```python
from build123d import *

# Parameters (mm, degrees)
BOSS_EXTRUDE1_DEPTH = 8
SKETCH2_W           = 23.137445614
SKETCH2_H           = 10.306738945
BOSS_EXTRUDE2_DEPTH = 8
SKETCH4_W           = 1
SKETCH4_H           = 2
CUT_EXTRUDE1_DEPTH  = 60
FILLET1_R           = 0.5


with BuildPart() as part:
    # Sketch1 → Boss-Extrude1 (new body)
    with BuildSketch(Plane(origin=(0, 0, 0), x_dir=(1, 0, 0), z_dir=(0, 1, 0))):
        with BuildLine():
            Line((11.568722807, -17.464704369), (11.568722807, 17.464704369))
            Line((11.568722807, 17.464704369), (0, 17.464704369))
            Line((0, 17.464704369), (0, -2.002357687))
            ThreePointArc((0, -2.002357687), (4.242640687, -3.759717), (6, -8.002357687))
            ThreePointArc((6, -8.002357687), (4.242640687, -12.244998375), (0, -14.002357687))
            Line((0, -14.002357687), (0, -17.464704369))
            Line((0, -17.464704369), (11.568722807, -17.464704369))
        make_face()
        with BuildLine():
            Line((0, -2.002357687), (0, 17.464704369))
            Line((0, 17.464704369), (-11.568722807, 17.464704369))
            Line((-11.568722807, 17.464704369), (-11.568722807, -17.464704369))
            Line((-11.568722807, -17.464704369), (0, -17.464704369))
            Line((0, -17.464704369), (0, -14.002357687))
            ThreePointArc((0, -14.002357687), (-6, -8.002357687), (0, -2.002357687))
        make_face()
    extrude(amount=BOSS_EXTRUDE1_DEPTH)

    # Sketch2 → Boss-Extrude2 (add)
    with BuildSketch(Plane.XZ):
        with Locations((0, -22.618073841)):
            Rectangle(SKETCH2_W, SKETCH2_H)
    extrude(amount=-BOSS_EXTRUDE2_DEPTH)

    # Sketch4 → Cut-Extrude1 (cut)
    with BuildSketch(Plane(origin=(11.568722807, 0, 0), x_dir=(0, 0, -1), z_dir=(1, 0, 0))):
        with Locations((13.536168456, 8)):
            Rectangle(SKETCH4_W, SKETCH4_H)
    extrude(amount=-CUT_EXTRUDE1_DEPTH, mode=Mode.SUBTRACT)

    # Fillet1
    fillet1_edges = [part.edges().sort_by_distance(p)[0] for p in [
        (0, 7, -14.036168456),
        (0, 7, -13.036168456),
    ]]
    fillet(fillet1_edges, radius=FILLET1_R - 0.0001)  # a hair under: the kernel refuses the full size


solid = part.part
```
Here's how the part is built. I have some questions about the finished solid (model axes, mm). Give positions to 0.01 mm unless a question says otherwise; leave off trailing zeros. Loops run counter-clockwise (first coordinate to the right, second up) from the corner with the lowest first, then second, coordinate; pieces in that order, holes last. Notation, with made-up numbers: M 83.25,-17 L 88.25,-17 A24 cw 88.25,5 Z; hole C 68,2 d5. An arc over 180 degrees is marked long. Use one line per item in the form item = value. Start each with the question number.
Q1. I need wall thicknesses on line 1 along Z through (x, y) = (-4.5, 4.75); line 2 along Z through (x, y) = (-2.75, 2.75); line 3 along X through (y, z) = (2.5, 7). Which ranges of each line are inside material? Lowest first, please.
Q2. If we section it at A-A (y = 6): Write out the boundary of the cut face in (x, z).
Q3. If we section it at B-B (z = 9): Write out the boundary of the cut face in (x, y).
Taken from the geometry:
q1.line_1 = -27.77 to 4.03, 11.97 to 17.46
q1.line_2 = -27.77 to 2.67, 13.34 to 17.46
q1.line_3 = -11.57 to -5.92, 5.92 to 11.57
q2.outline = M -11.57,-27.77 L 11.57,-27.77 L 11.57,17.46 L -11.57,17.46 Z; hole C 0,8 d12
q3.outline = M -11.57,0 L -5.92,0 L -5.92,8 L -11.57,8 Z; M 5.92,0 L 11.57,0 L 11.57,8 L 5.92,8 Z
